Geometry check sheet. Reference: the model listing, model coordinates, mm. A direction names the side the tool comes from. Round coordinates to 2 decimals unless told otherwise and drop trailing zeros. Order: outer loops, then holes, each group sorted by start corner. A loop starts at its lowest first (then second) coordinate and runs counter-clockwise, first axis right, second up.
(1) Sectioned sample at C-C (y = 313.5). Record the boundary of the cut face in (x, z).
(2) Material ranges on line 1 along X through (y, z) = (275.3, -1.3); line 2 along X through (y, z) = (282, -43.5); line 3 along Z through (x, y) = (59, 308.5), recorded low to high.
(3) Release check for a two-part mould opening along X. For faces 4 (the face through (-52, 302, -4)), 5 (the face through (38.5, 302, -32)), 6 (the face through (58.87, 327.47, -1.97)), 7 (the face through (-56.13, 327.47, -1.97)) record: +X half, -X half, draft (parallel to the pull), parting line (faces both ways), or undercut.
(4) Sectioned sample at A-A (y = 330.3). Record the boundary of the cut face in (x, z), plus the area to 3 significant figures.
(5) Set-up check for faces 1 (the face through (-32, 302, -26)), 2 (the face through (54, 302, -4)), 3 (the face through (-38.5, 302, -33)): record each of +Z, -Z, +X, -X, +Y, -Y from which the full face is reachable in a straight line by a thin tool's end or side.
(6) Go/stop test with flat-tipped pins: pin 1 (1 mm diameter, centred on y = 274, z = -9.5, fed in from -X); pin 2 (3 mm diameter, centred on y = 315, z = -40, fed in from +X); pin 3 (8 mm diameter, centred on x = -0.5, y = 320, fed in from +Z). Record where each tip stops, or that it passes through.
(7) Sectioned sample at D-D (x = -25). Record the boundary of the cut face in (y, z), plus the area to 3 significant figures.
(8) Sectioned sample at B-B (z = -38.5). Record the boundary of the cut face in (x, y).
from build123d import *

# Parameters (mm, degrees)
PAD002_DEPTH   = 75
SKETCH006_R    = 2.9
HOLE002_DEPTH  = 25
HOLE002_TIPS_R = 2.9


with BuildPart() as part:
    # Sketch005 → Pad002 (new body)
    with BuildSketch(Plane.XZ):
        Polygon((-38, 0), (-0.5, 0), (-0.5, -4), (-31.5, -4), (-31.5, -60.5), (-108.5, -60.5), (-108.5, -4), (-135, -4), (-135, 0), (-102, 0), (-102, -52.5), (-38, -52.5), align=None)
    extrude(amount=-PAD002_DEPTH)

    # Sketch006 → Hole002 (cut)
    with BuildSketch(Plane.XY):
        with Locations((-125.500002, 10.3)):
            Circle(SKETCH006_R)
        with Locations((-125.500002, 65.3)):
            Circle(SKETCH006_R)
        with Locations((-10.500002, 10.3)):
            Circle(SKETCH006_R)
        with Locations((-10.500002, 65.3)):
            Circle(SKETCH006_R)
    extrude(amount=-HOLE002_DEPTH, mode=Mode.SUBTRACT)

    # Hole002 tips → Hole002 tip 1 section 0
    with BuildSketch(Plane.XY.offset(-25), mode=Mode.PRIVATE) as hole002_tip_1_s0:
        with Locations((-125.500002, 10.3)):
            Circle(HOLE002_TIPS_R)
    loft([hole002_tip_1_s0.sketch, Vertex(-125.500002, 10.3, -26.742496)], mode=Mode.SUBTRACT)

    # Hole002 tips → Hole002 tip 2 section 0
    with BuildSketch(Plane.XY.offset(-25), mode=Mode.PRIVATE) as hole002_tip_2_s0:
        with Locations((-125.500002, 65.3)):
            Circle(HOLE002_TIPS_R)
    loft([hole002_tip_2_s0.sketch, Vertex(-125.500002, 65.3, -26.742496)], mode=Mode.SUBTRACT)

    # Hole002 tips → Hole002 tip 3 section 0
    with BuildSketch(Plane.XY.offset(-25), mode=Mode.PRIVATE) as hole002_tip_3_s0:
        with Locations((-10.500002, 10.3)):
            Circle(HOLE002_TIPS_R)
    loft([hole002_tip_3_s0.sketch, Vertex(-10.500002, 10.3, -26.742496)], mode=Mode.SUBTRACT)

    # Hole002 tips → Hole002 tip 4 section 0
    with BuildSketch(Plane.XY.offset(-25), mode=Mode.PRIVATE) as hole002_tip_4_s0:
        with Locations((-10.500002, 65.3)):
            Circle(HOLE002_TIPS_R)
    loft([hole002_tip_4_s0.sketch, Vertex(-10.500002, 65.3, -26.742496)], mode=Mode.SUBTRACT)


with BuildPart() as part_1:
    # Body002 placement: moved
    add(part.part.moved(Location((70, 265, 0))))


solid = part_1.part
Answer below:
1. outline: (-65, -4) - (-38.5, -4) - (-38.5, -60.5) - (38.5, -60.5) - (38.5, -4) - (69.5, -4) - (69.5, 0) - (32, 0) - (32, -52.5) - (-32, -52.5) - (-32, 0) - (-65, 0) - close
2. line 1: x = -65 to -58.4, -52.6 to -32, 32 to 56.6, 62.4 to 69.5
2. line 2: x = -38.5 to -32, 32 to 38.5
2. line 3: z = -4 to 0
3. face 4: draft
3. face 5: +X half
3. face 6: undercut
3. face 7: undercut
4. outline: (-65, -4) - (-58.4, -4) - (-58.4, 0) - (-65, 0) - close; (-52.6, -4) - (-38.5, -4) - (-38.5, -60.5) - (38.5, -60.5) - (38.5, -4) - (56.6, -4) - (56.6, 0) - (32, 0) - (32, -52.5) - (-32, -52.5) - (-32, 0) - (-52.6, 0) - close; (62.4, -4) - (69.5, -4) - (69.5, 0) - (62.4, 0) - close
4. area: 1,480 mm2
5. face 1: +Z, +Y, -Y
5. face 2: -Z, +X, +Y, -Y
5. face 3: -Z, -X, +Y, -Y
6. pin 1: stops at x = -38.5
6. pin 2: stops at x = 38.5
6. pin 3: stops at z = -52.5
7. outline: (265, -60.5) - (340, -60.5) - (340, -52.5) - (265, -52.5) - close
7. area: 600 mm2
8. outline: (-38.5, 265) - (-32, 265) - (-32, 340) - (-38.5, 340) - close; (32, 265) - (38.5, 265) - (38.5, 340) - (32, 340) - close
